from build123d import *

# Parameters (mm, degrees)
REVOLVE1_ANGLE             = 35
CUT_EXTRUDE1_DEPTH         = 12.7
CUT_EXTRUDE2_DEPTH         = 12.7
F_9_0_196_DIAMETER_HOLE1_D = 4.9784


with BuildPart() as part:
    # Sketch1 → Revolve1 (revolve)
    with BuildSketch(Plane(origin=(0, 0, 0), x_dir=(0, 1, 0), z_dir=(0, 0, 1))):
        with BuildLine():
            Line((0, 0), (0, 25.4))
            Line((0, 25.4), (-19.05, 25.4))
            ThreePointArc((-19.05, 25.4), (-14.199031657, 12.7), (-19.05, 0))
            Line((-19.05, 0), (0, 0))
        make_face()
    revolve(axis=Axis((-25.4, 169.5196, 0), (1, 0, 0)), revolution_arc=REVOLVE1_ANGLE)

    # Sketch2 → Cut-Extrude1 (cut)
    with BuildSketch(Plane.YZ):
        with BuildLine():
            Line((-19.05, 0), (169.5196, 0))
            Line((169.5196, 0), (-18.332435741, -16.434923548))
            ThreePointArc((-18.332435741, -16.434923548), (-18.870523524, -8.225290428), (-19.05, 0))
        make_face()
    extrude(amount=-CUT_EXTRUDE1_DEPTH, mode=Mode.SUBTRACT)

    # Sketch3 → Cut-Extrude2 (cut)
    with BuildSketch(Plane(origin=(-25.4, 0, 0), x_dir=(0, -1, 0), z_dir=(-1, 0, 0))):
        with BuildLine():
            Line((-15.052426669, -108.159079172), (-169.5196, 0))
            Line((-169.5196, 0), (-6.213536019, -94.2848))
            ThreePointArc((-6.213536019, -94.2848), (-10.48161242, -101.318372226), (-15.052426669, -108.159079172))
        make_face()
    extrude(amount=-CUT_EXTRUDE2_DEPTH, mode=Mode.SUBTRACT)

    # #9 (0.196) Diameter Hole1 (through all)
    with Locations(Plane.YZ):
        with Locations((22.799344486, -93.471111446), (-4.279424248, -7.588229275)):
            Hole(F_9_0_196_DIAMETER_HOLE1_D / 2)


solid = part.part
Check sheet for the modelled part. Datum: model origin and axes. Units: mm. A direction names the side the tool comes from. Give positions to 0.01 mm unless a question says otherwise; leave off trailing zeros. Order: outer loops, then holes, each group sorted by start corner. A loop starts at its lowest first (then second) coordinate and runs counter-clockwise, first axis right, second up. Notation, with made-up numbers: M -23,4.5 L -18,4.5 A27 cw -18,37.5 Z; hole C -13.75,-8 d10. An arc over 180 degrees is marked long. Answer as CSV lines item,"result". Start each with the question number.
Item 1: Tool access check on faces 4 (the face through (-6.26, -6.6, -15.41)), 5 (the face through (-6.44, 21.65, -95.68)), 6 (the face through (-12.7, 20, -95)). Record the directions out of +Z, -Z, +X, -X, +Y, -Y that give a thin tool (end or side, any length) a straight path to the whole face; none if there is none.
Item 2: Mould release check, pull along Z, two halves, no side actions. Record for faces 1 (the face through (-12.88, 7.63, -50.28)), 2 (the face through (-25.4, -3, -48)), 3 (the face through (-19.14, -3.74, -10.02)): +Z half, -Z half, draft (parallel to the pull), parting line (faces both ways), or undercut.
Item 3: Cross-section at A-A on x = -15.75. Enter the section's corners in (y, z).
Item 4: Gauge pin test, flat ends, axial feed: P1, Ø4.5, axis at y = -6, z = -9, coming from the +X side; P2, Ø10, axis at x = -6, z = -69, coming from the -Y side; P3, Ø5, axis at x = -5.5, z = -85, coming from the +Y side. Record the tip position at first contact, or that the pin passes through.
Item 5: Thickness scan on line 1 (X direction, y = -13, z = -6.5); line 2 (X direction, y = 5, z = -89); line 3 (X direction, y = 20, z = -94). Record the ranges inside material, lowest first. Write a range as [from, to].
Item 6: Cross-section at B-B on x = -22. Enter the section's corners in (y, z).
Established:
1,face 4,"+Z, +X, -Y"
1,face 5,"+X, -X"
1,face 6,"-Z, -X, +Y"
2,face 1,"+Z half"
2,face 2,"draft"
2,face 3,"undercut"
3,outline,"M -14.44,0 A183.96 ccw 10.2,-91.98 L 22.71,-84.76 A169.52 cw 0,0 Z; hole C -4.28,-7.59 d4.98"
4,P1,"stops at x = -12.7"
4,P2,"stops at y = -5.52"
4,P3,"stops at y = 24.33"
5,line 1,"x = [-25.4, -12.7]"
5,line 2,"x = [-25.4, -23.46], [-1.94, 0]"
5,line 3,"x = [-12.7, 0]"
6,outline,"M -16.62,0 A186.14 ccw 8.32,-93.07 L 22.71,-84.76 A169.52 cw 0,0 Z; hole C -4.28,-7.59 d4.98"
